Verification items for the finished model (mm, model axes). Round coordinates to 2 decimals unless told otherwise and drop trailing zeros. Loops run counter-clockwise (first coordinate to the right, second up) from the corner with the lowest first, then second, coordinate; pieces in that order, holes last. Notation, with made-up numbers: (72, -5) -> (130, -5) arc R17 ccw to (130, 18) -> close; hole circle Ø2 at (35, -40). An arc over 180 degrees is marked (long way). Use CSV: the item, a comma, the result in double quotes. Start each with the question number.
```python
from build123d import *

# Parameters (mm, degrees)
SKETCH2_R           = 6.35
BOSS_EXTRUDE1_DEPTH = 5.08


with BuildPart() as part:
    # Sketch2 → Boss-Extrude1 (new body)
    with BuildSketch(Plane(origin=(0, 0, 0), x_dir=(1, 0, 0), z_dir=(0, 1, 0))):
        with BuildLine():
            Line((-595.5, -12.7), (0, -12.7))
            ThreePointArc((0, -12.7), (12.7, 0), (0, 12.7))
            Line((0, 12.7), (-340.965168315, 30.430994835))
            ThreePointArc((-340.965168315, 30.430994835), (-341.544922169, 30.443467581), (-342.124360605, 30.420637788))
            Line((-342.124360605, 30.420637788), (-595.5, 12.7))
            ThreePointArc((-595.5, 12.7), (-608.2, 0), (-595.5, -12.7))
        make_face()
        with Locations(Location((0, 0, 0), (0, 0, 270))):
            Circle(SKETCH2_R, mode=Mode.SUBTRACT)
        with Locations(Location((-595.5, 0, 0), (0, 0, 270))):
            Circle(SKETCH2_R, mode=Mode.SUBTRACT)
        with Locations(Location((-341.459822451, 20.918847744, 0), (0, 0, 270))):
            Circle(SKETCH2_R, mode=Mode.SUBTRACT)
    extrude(amount=-BOSS_EXTRUDE1_DEPTH)


solid = part.part
```
Q1. Release check for a two-part mould opening along Z. For faces 1 (the face through (-335.164, -2.504, -21.745)), 2 (the face through (-608.197, -2.504, -0.279)), 3 (the face through (-302, 0, -4)) record: +Z half, -Z half, draft (parallel to the pull), parting line (faces both ways), or undercut.
Q2. Depth check by flat-ended pin: pin 1 Ø1.5 at (y, z) = (-2, -9.5) entering from -X; pin 2 Ø1.5 at (y, z) = (-4.5, 4) entering from +X; pin 3 Ø7.5 at (x, z) = (-341.46, -20.92) entering from +Y. Enter the tip coordinate at first touch or a pass-through.
Q3. Thickness scan on L1, parallel to X at y = -3.9, z = 0; L2, parallel to X at y = -4.5, z = -1.5; L3, parallel to Z at x = -595.5, y = -1.5. Record the ranges inside material, lowest first. Write a range as from..to.
Q4. Cross-section at D-D (x = -143). Record the boundary of the cut face in (y, z).
Q5. Cross-section at A-A (z = 0). Record the boundary of the cut face in (x, y).
Q6. Cross-section at C-C (x = -496). Record the boundary of the cut face in (y, z).
Q7. Cross-section at B-B (y = -1.2). Record the boundary of the cut face in (x, z) (3 decimals).
Answer list:
1,face 1,"undercut"
1,face 2,"parting line"
1,face 3,"draft"
2,pin 1,"stops at x = -604.7"
2,pin 2,"stops at x = 12.28"
2,pin 3,"passes through"
3,L1,"x = -608.2..-601.85, -589.15..-6.35, 6.35..12.7"
3,L2,"x = -608.11..-601.67, -589.33..-6.17, 6.17..12.61"
3,L3,"z = -12.7..-6.35, 6.35..12.7"
4,outline,"(-5.08, -20.14) -> (0, -20.14) -> (0, 12.7) -> (-5.08, 12.7) -> close"
5,outline,"(-608.2, -5.08) -> (-601.85, -5.08) -> (-601.85, 0) -> (-608.2, 0) -> close; (-589.15, -5.08) -> (-6.35, -5.08) -> (-6.35, 0) -> (-589.15, 0) -> close; (6.35, -5.08) -> (12.7, -5.08) -> (12.7, 0) -> (6.35, 0) -> close"
6,outline,"(-5.08, -19.66) -> (0, -19.66) -> (0, 12.7) -> (-5.08, 12.7) -> close"
7,outline,"(-595.5, -12.7) -> (-342.124, -30.421) arc R9.525 ccw to (-340.965, -30.431) -> (0, -12.7) arc R12.7 ccw to (0, 12.7) -> (-595.5, 12.7) arc R12.7 ccw to start; hole circle Ø12.7 at (-595.5, 0); hole circle Ø12.7 at (-341.46, -20.919); hole circle Ø12.7 at (0, 0)"
